Can you work these out from the model? Positions are in its coordinate system, mm. A direction names the side the tool comes from. Coordinates: 2 decimals unless noted, no trailing zeros. Order: outer loops, then holes, each group sorted by start corner. A loop starts at its lowest first (then second) coordinate and runs counter-clockwise, first axis right, second up. Notation, with made-up numbers: (-17, -14) -> (16, -14) arc R22 cw to (16, -6) -> close; hole circle Ø9 at (-27, 60.5). An arc over 180 degrees is marked (long way). Return JSON: item names as keys, results as strings. Group by question number.
1) If we section it at A-A, the plane y = 8: Please give me the cut outline in (x, z), then the cut area to 3 significant figures.
2) If I drill on probe 1 along X at (y, z) = (15.75, 16.25); probe 2 along X at (y, z) = (4.5, 10); probe 3 along Z at (x, y) = (3.6, 20.5), over which ranges is the centre line in solid material (lowest first)? Write a range as from..to.
3) If we section it at B-B, the plane y = 20.5: Please give me the cut outline in (x, z), then the cut area to 3 significant figures.
4) Thinking about a two-plate mould opening in Z: for faces 4 (the cylindrical face through (11.9, 4.22, 9.53)), 5 (the flat face through (0, 15, 10)), 6 (the cylindrical face through (25.042, 27.594, 2.281)), which applies, +Z half, -Z half, draft (parallel to the pull), parting line (faces both ways), or undercut?
5) If we section it at C-C, the plane z = 10: State how many separate pieces and enclosed holes the cut face has, then the cut area to 3 significant figures.
6) For pin 1 (8 mm diameter, centred on x = 10.5, z = 14, fed in from +Y), with a flat end and sliding along its axis, tell me the tip position at first contact or that it passes through.
7) For faces 1 (the flat face through (6, 17.8, 10.1)), 2 (the flat face through (14, 0, 12)), 3 (the flat face through (12, 3, 10)), which set-ups out of +Z, -Z, +X, -X, +Y, -Y let a thin tool reach every point of the face, with its end or its side?
from build123d import *

# Parameters (mm, degrees)
SKETCH1_W               = 28
SKETCH1_H               = 20
BOSS_EXTRUDE1_DEPTH     = 6
SKETCH2_W               = 6
SKETCH2_H               = 20
BOSS_EXTRUDE2_DEPTH     = 24
CUT_EXTRUDE1_DEPTH      = 43.237424164
CUT_EXTRUDE1_DEPTH_BACK = 43.237424164
SKETCH3_R               = 2.45
SKETCH4_R               = 1.65
CUT_EXTRUDE2_DEPTH      = 42.952353927
SKETCH5_R               = 2.15
CUT_EXTRUDE3_DEPTH      = 3
FILLET1_SIZE            = 0.6
FILLET2_R               = 8


with BuildPart() as part:
    # Sketch1 → Boss-Extrude1 (new body)
    with BuildSketch(Plane(origin=(0, 0, 0), x_dir=(1, 0, 0), z_dir=(0, 1, 0))):
        with Locations((14, -10)):
            Rectangle(SKETCH1_W, SKETCH1_H)
    extrude(amount=BOSS_EXTRUDE1_DEPTH)

    # Sketch2 → Boss-Extrude2 (add)
    with BuildSketch(Plane(origin=(0, 6, 0), x_dir=(1, 0, 0), z_dir=(0, 1, 0))):
        with Locations((3, -10)):
            Rectangle(SKETCH2_W, SKETCH2_H)
        with Locations((25, -10)):
            Rectangle(SKETCH2_W, SKETCH2_H)
    extrude(amount=BOSS_EXTRUDE2_DEPTH)

    # Sketch3 → Cut-Extrude1 (cut, two sides: drawn at the far end of the back side and taken through both)
    with BuildSketch(Plane(origin=(6, 0, 0), x_dir=(0, 0, -1), z_dir=(1, 0, 0)).offset(-CUT_EXTRUDE1_DEPTH_BACK)):
        with Locations((-10, 20.5)):
            Circle(SKETCH3_R)
    extrude(amount=CUT_EXTRUDE1_DEPTH + CUT_EXTRUDE1_DEPTH_BACK, mode=Mode.SUBTRACT)

    # Sketch4 → Cut-Extrude2 (cut, through all)
    with BuildSketch(Plane(origin=(0, 6, 0), x_dir=(1, 0, 0), z_dir=(0, 1, 0))):
        with Locations(Location((14, -10, 0), (0, 0, 270))):
            Circle(SKETCH4_R)
    extrude(amount=-CUT_EXTRUDE2_DEPTH, mode=Mode.SUBTRACT)

    # Sketch5 → Cut-Extrude3 (cut)
    with BuildSketch(Plane(origin=(0, 6, 0), x_dir=(1, 0, 0), z_dir=(0, 1, 0))):
        with Locations(Location((14, -10, 0), (0, 0, 270))):
            Circle(SKETCH5_R)
    extrude(amount=-CUT_EXTRUDE3_DEPTH, mode=Mode.SUBTRACT)

    # Fillet1
    # a fillet whose section is not a circle: 0.6 mm, written as the material it takes off along each edge
    with BuildSketch(Plane(origin=(14, 6, 10), x_dir=(0, 0, 1), z_dir=(-1, 0, 0))) as fillet1_piece_1:
        with BuildLine():
            Bezier((2.15 + FILLET1_SIZE, 0), (2.15, 0), (2.15, -FILLET1_SIZE), weights=[1, 0.052631579, 1])
            Line((2.15, -FILLET1_SIZE), (2.15, 0))
            Line((2.15, 0), (2.15 + FILLET1_SIZE, 0))
        make_face()
    revolve(axis=Axis((14, 6, 10), (0, 1, 0)), mode=Mode.SUBTRACT)

    # Fillet2
    fillet2_edges = [part.edges().sort_by_distance(p)[0] for p in [
        (3, 30, 20),
        (3, 30, 0),
        (25, 30, 0),
        (25, 30, 20),
    ]]
    fillet(fillet2_edges, radius=FILLET2_R)


solid = part.part
Result sheet:
{
 "1": {"outline": "(0, 0) -> (6, 0) -> (6, 20) -> (0, 20) -> close; (22, 0) -> (28, 0) -> (28, 20) -> (22, 20) -> close", "area": "240 mm2"},
 "2": {"probe 1": "x = 0..6, 22..28", "probe 2": "x = 0..11.85, 16.15..28", "probe 3": "z = 0..7.55, 12.45..20"},
 "3": {"outline": "(0, 0) -> (6, 0) -> (6, 7.55) -> (0, 7.55) -> close; (0, 12.45) -> (6, 12.45) -> (6, 20) -> (0, 20) -> close; (22, 0) -> (28, 0) -> (28, 7.55) -> (22, 7.55) -> close; (22, 12.45) -> (28, 12.45) -> (28, 20) -> (22, 20) -> close", "area": "181 mm2"},
 "4": {"face 4": "undercut", "face 5": "draft", "face 6": "-Z half"},
 "5": {"separate pieces": "4", "enclosed holes": "0", "area": "374 mm2"},
 "6": {"pin 1": "stops at y = 6"},
 "7": {"face 1": "+Z, -Z, +Y", "face 2": "+Z, -Z, +X, -X, -Y", "face 3": "+Y"}
}
